For this review, take the finished solid that the model builds, in its own axes (mm). Coordinates: 2 decimals unless noted, no trailing zeros. Loops run counter-clockwise (first coordinate to the right, second up) from the corner with the lowest first, then second, coordinate; pieces in that order, holes last. Notation, with made-up numbers: (31, 31) - (47, 31) arc R28 cw to (47, 61) - close; hole circle Ø4 at (-36.5, 33.5). An arc over 180 degrees is marked (long way). Answer as a JSON object with one key per item and string values. Group by question number.
Item 1: We need section C-C (y = 36). Give the boundary of the cut face in (x, z), then the cut area to 3 significant figures.
Item 2: To check wall thickness, follow line 1 (Y direction, x = 18, z = -36); line 2 (X direction, y = 39, z = -5); line 3 (Z direction, x = 38, y = 57.5). State the ranges of each line that lie inside material, in increasing order.
Item 3: We need section B-B (z = -48.5). Give the boundary of the cut face in (x, y).
Item 4: Clearance check with flat-ended pins moving along their axes: pin 1 (6 mm diameter, centred on x = 35, y = 38.5, fed in from -Z); pin 2 (12 mm diameter, centred on x = 25, y = 10.5, fed in from +Z); pin 3 (10 mm diameter, centred on x = 15, z = -30.5, fed in from +Y). State where each tip first meets the part, or that it passes through.
Item 5: We need section A-A (x = 37.5). Give the boundary of the cut face in (y, z), then the cut area to 3 significant figures.
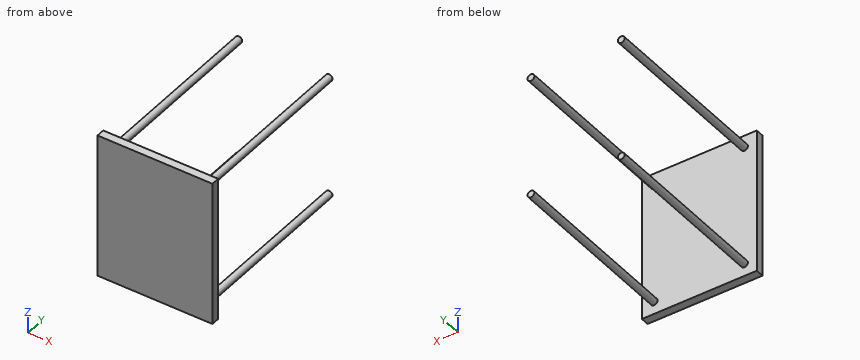
Autodesk Inventor part; units mm, degrees
ref_plane "YZ Plane" through (0, 0, 0) normal (1, 0, 0) x (0, 1, 0)
ref_plane "XZ Plane" through (0, 0, 0) normal (0, 1, 0) x (-1, 0, 0)
ref_plane "XY Plane" through (0, 0, 0) normal (0, 0, 1) x (1, 0, 0)
sketch "Boceto1" plane through (0, 0, 0) normal (0, 1, 0) x (-1, 0, 0)
  line L0 (0, 0) -> (-42, 0)
  line L1 (-42, 0) -> (-42, -53)
  line L2 (-42, -53) -> (0, -53)
  line L3 (0, -53) -> (0, 0)
  circle A0 centre (-4.5, -4.5) radius 1.25
  circle A1 centre (-4.5, -48.5) radius 1.25
  circle A2 centre (-37.5, -48.5) radius 1.25
  circle A3 centre (-37.5, -4.5) radius 1.25
  line L4 (-36.25, -48.5) -> (-5.75, -48.5)
  line L5 (-4.5, -47.25) -> (-4.5, -5.75)
  line L6 (-5.75, -4.5) -> (-36.25, -4.5)
  line L7 (-37.5, -5.75) -> (-37.5, -47.25)
  dimension "d0" = 42
  dimension "d1" = 53
  dimension "d2" = 2.5
  dimension "d4" = 2.5
  dimension "d6" = 2.5
  dimension "d7" = 2.5
extrude "Extrusión1" add sketch "Boceto1" along normal blind 3 contours L3 L2 L1 L0 | A0 | A0 L5 A1 L4 A2 L7 A3 L6 | A3 | A1 | A2
sketch "Boceto2" plane through (0, 3, 0) normal (0, 1, 0) x (1, 0, 0)
  circle A0 centre (4.5, 4.5) radius 1.25
  circle A1 centre (4.5, 4.5) radius 1.25
  circle A2 centre (4.5, 48.5) radius 1.25
  circle A3 centre (4.5, 48.5) radius 1.25
  circle A4 centre (37.5, 48.5) radius 1.25
  circle A5 centre (37.5, 48.5) radius 1.25
  circle A6 centre (37.5, 4.5) radius 1.25
  circle A7 centre (37.5, 4.5) radius 1.25
  point P0 (0, 0)
extrude "Extrusión2" add sketch "Boceto2" along normal blind 65
properties part number "Relé - columnes"
Check sheet entries:
{
 "1": {"outline": "circle Ø2.5 at (4.5, -48.5); circle Ø2.5 at (4.5, -4.5); circle Ø2.5 at (37.5, -48.5); circle Ø2.5 at (37.5, -4.5)", "area": "19.6 mm2"},
 "2": {"line 1": "y = 0 to 3", "line 2": "x = 3.35 to 5.65, 36.35 to 38.65", "line 3": "z = -49.65 to -47.35, -5.65 to -3.35"},
 "3": {"outline": "(0, 0) - (42, 0) - (42, 3) - (38.75, 3) - (38.75, 68) - (36.25, 68) - (36.25, 3) - (5.75, 3) - (5.75, 68) - (3.25, 68) - (3.25, 3) - (0, 3) - close"},
 "4": {"pin 1": "stops at z = -49.75", "pin 2": "passes through", "pin 3": "stops at y = 3"},
 "5": {"outline": "(0, -53) - (3, -53) - (3, -49.75) - (68, -49.75) - (68, -47.25) - (3, -47.25) - (3, -5.75) - (68, -5.75) - (68, -3.25) - (3, -3.25) - (3, 0) - (0, 0) - close", "area": "484 mm2"}
}
